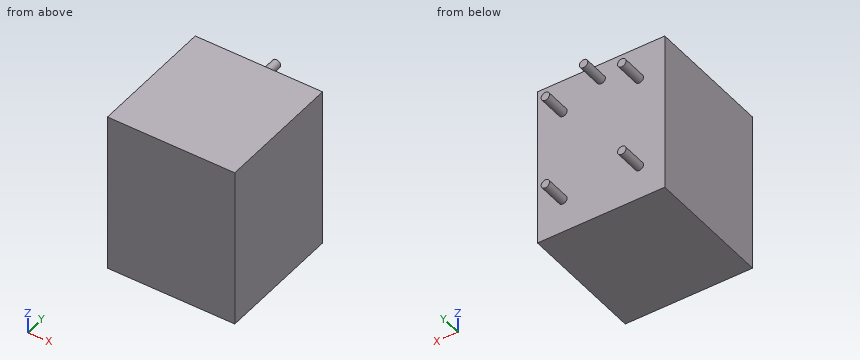
Autodesk Inventor part; units mm, degrees
ref_plane "YZ Plane" through (0, 0, 0) normal (1, 0, 0) x (0, 1, 0)
ref_plane "XZ Plane" through (0, 0, 0) normal (0, 1, 0) x (-1, 0, 0)
ref_plane "XY Plane" through (0, 0, 0) normal (0, 0, 1) x (1, 0, 0)
sketch "Sketch1" plane through (0, 0, 0) normal (0, 1, 0) x (-1, 0, 0)
  line L0 (0, 0) -> (15, 0)
  line L1 (15, 0) -> (15, -19)
  line L2 (15, -19) -> (0, -19)
  line L3 (0, -19) -> (0, 0)
  dimension "d0" = 19
  dimension "d1" = 15
extrude "Extrusion1" add sketch "Sketch1" along normal blind 15
sketch "Sketch2" plane through (0, 15, 0) normal (0, 1, 0) x (1, 0, 0)
  circle A0 centre (-3, 4) radius 0.5
  line L0 (0, 0) -> (0, 19)
  line L1 (-15, 0) -> (0, 0)
  circle A1 centre (-3, 15) radius 0.5
  line L2 (0, 19) -> (-15, 19)
  circle A2 centre (-7.5, 2) radius 0.5
  line L3 (-7.5, 0) -> (-7.5, 19) construction
  circle A3 centre (-12, 4) radius 0.5
  circle A4 centre (-12, 15) radius 0.5
  dimension "d4" = 1
  dimension "d5" = 3
  dimension "d6" = 4
  dimension "d7" = 1
  dimension "d8" = 3
  dimension "d9" = 4
  dimension "d10" = 1
  dimension "d11" = 2
extrude "Extrusion2" add sketch "Sketch2" along normal blind 3
sketch "Sketch3" plane through (-12, 18, -4) normal (0, 1, 0) x (1, 0, 0)
  circle A0 centre (4.5, -2) radius 0.5
  circle A1 centre (9, 0) radius 0.5
  circle A2 centre (9, 11) radius 0.5
  circle A3 centre (0, 0) radius 0.5
  circle A4 centre (0, 11) radius 0.5
  point P0 (12, -4)
properties part number "miniRelay"
Source: CAD feature listing. Evaluate the final solid. Frame: model axes, mm. Round coordinates to 2 decimals unless told otherwise and drop trailing zeros. Loops run counter-clockwise (first coordinate to the right, second up) from the corner with the lowest first, then second, coordinate; pieces in that order, holes last.
1. Section query B-B on x = -3. Output: boundary loops of the cut face in (y, z).
2. Section query A-A on z = -4. Output: boundary loops of the cut face in (x, y), and give its area (3 significant figures).
3. Contact query for flat-ended pins moving along their axis: pin 1 (3 mm diameter, centred on y = 8, z = -5.5, fed in from +X); pin 2 (7.5 mm diameter, centred on x = -7, z = -10, fed in from +Y). Output: stop coordinate, or through.
4. Ray query, L1, parallel to Y at x = -5.5, z = -14.75. Return the intervals inside material, ascending.
5. Section query C-C on z = -2. Output: boundary loops of the cut face in (x, y).
6. Section query D-D on x = -6.25. Output: boundary loops of the cut face in (y, z).
Answers below:
1. outline: (0, -19) - (15, -19) - (15, -15.5) - (18, -15.5) - (18, -14.5) - (15, -14.5) - (15, -4.5) - (18, -4.5) - (18, -3.5) - (15, -3.5) - (15, 0) - (0, 0) - close
2. outline: (-15, 0) - (0, 0) - (0, 15) - (-2.5, 15) - (-2.5, 18) - (-3.5, 18) - (-3.5, 15) - (-11.5, 15) - (-11.5, 18) - (-12.5, 18) - (-12.5, 15) - (-15, 15) - close
2. area: 231 mm2
3. pin 1: stops at x = 0
3. pin 2: stops at y = 15
4. L1: y = 0 to 15
5. outline: (-15, 0) - (0, 0) - (0, 15) - (-7, 15) - (-7, 18) - (-8, 18) - (-8, 15) - (-15, 15) - close
6. outline: (0, -19) - (15, -19) - (15, 0) - (0, 0) - close
